Part model, mm, in its own coordinate system. A direction names the side the tool comes from. Give positions to 0.01 mm unless a question says otherwise; leave off trailing zeros. Write each loop counter-clockwise with the first axis right and the second up, starting at its lowest first coordinate (ties: lowest second). Pieces come first, ordered by that corner, then holes. Notation, with made-up numbers: M 69,15 L 81,15 A29 cw 81,48 Z; hole C -40,23 d11. An arc over 180 degrees is marked long. Use CSV: the item, a comma, the result in double quotes. Start each with the question number.
Item 1: Cut at A-A (z = 5). List the corners of the cut face in (x, y), then the cut area to 3 significant figures.
Item 2: Which spindle directions (+Z, -Z, +X, -X, +Y, -Y) get a long thin tool onto all of the face, cutting with end or side? Do faces 1 (the cylindrical face through (-69.244, -24.742, 7.365)), 2 (the flat face through (67, 46, 65.404)), 3 (the cylindrical face through (26.19, 75.94, 61.1)). Say none if no direction does.
Item 3: Drill centre lines: line 1 (X direction, y = 0, z = 48); line 2 (X direction, y = 0, z = -5); line 3 (Z direction, x = 64, y = 49). Where is each one in solid material? Low to high. Write a range as [from, to].
Item 4: Mould opens along Y. For faces 4 (the conical face through (-66.956, 31.627, -42.848)), 5 (the cylindrical face through (-60.5, -22, 61.2)), 6 (the flat face through (9, -77, -45.591)) say: released by +Y, released by -Y, zero draft, split by the parting line, or undercut.
Item 5: Pin check, flat tips, straight feed: pin 1 (2 mm diameter, centred on y = 47, z = 33, fed in from -X); pin 2 (1.5 mm diameter, centred on x = 30.5, y = -52, fed in from -Z); pin 3 (1.5 mm diameter, centred on y = -53, z = 11.5, fed in from +X). Stop position of each tip, or through.
from build123d import *

# Parameters (mm, degrees)
F2_T            = 4.5
F4_DEPTH        = 2.5
F4_COPIES_COUNT = 4
F5_S5_R         = 5
F5_T6_DEPTH     = 125
F5_S7_R         = 5
F5_T8_DEPTH     = 125
F5_S9_R         = 5
F5_T10_DEPTH    = 125
F5_S11_R        = 5
F5_T12_DEPTH    = 125


# Not quite as in the source:
# - a fillet or chamfer that OpenCascade refuses, or shapes differently, is made with other operations: its cross-section is extruded or revolved along the edge and cut away or added
# - a pattern or mirror of a feature is missing from the dataset's text; its kind, count and spacing are read off the source's solid
# - a shell that OpenCascade refuses in one call is made with other operations: the cavity is built on its own and cut out


with BuildPart() as f1:
    # F0 (on Front) → F1 (revolve)
    with BuildSketch(Plane.XZ):
        Polygon((9.3241020494, -43.0905388618), (9.3241020494, 56.9094611382), (-63.8827484445, 56.9094611382), (-63.8827484445, 65.4041709328), (-68.4650088725, 65.4041709328), (-68.4650088725, 56.9094611382), (-73.0472693004, 56.9094611382), (-73.0472693004, 61.1568160355), (-75.6501782344, 61.1568160355), (-78.0099242383, 55.0157746972), (-78.0099242383, 40.8573164567), (-73.0472693004, 36.7660618934), (-73.0472693004, -21.2237248131), (-78.0099242383, -30.2868788943), (-78.0099242383, -43.0905388618), align=None)
    revolve(axis=Axis((9.3241020494, 0, 6.9094611382), (0, 0, 1)))

    # F2: shell of thickness 4.5, made by hand


with BuildPart() as f2_core1:
    # F2_t2: copy of F1
    add(f1.part)

    # the walls: a layer under each face that stays
    f2_faces = [f2_core1.faces().sort_by_distance(p)[0] for p in [
        (82.5309525433, 0, 61.1568160355),
        (-42.5353052318, 51.8594072813, 65.4041709328),
        (87.1132129713, 0, 61.1568160355),
        (-67.5558445438, 21.9656990266, 56.9094611382),
        (91.6954733993, 0, 59.0331385869),
        (-69.9852262155, 22.6598080757, 61.1568160355),
        (95.4782553352, 0, 58.0862953663),
        (96.6581283371, 0, 47.936545577),
        (94.1768008682, 0, 38.8116891751),
        (91.6954733993, 0, 7.7711685402),
        (94.1768008682, 0, -25.7553018537),
        (96.6581283371, 0, -36.688708878),
        (9.3241020494, 0, -43.0905388618),
    ]]
    thicken(f2_faces, amount=-F2_T, mode=Mode.SUBTRACT)

    # F2_s3 → F2_t4 (revolve, cut)
    with BuildSketch(Plane.XZ):
        Polygon((-68.5100088725, 56.9544611382), (-63.9650088725, 56.9094611382), (-63.9650088725, 52.4094611382), (-68.4650088725, 52.4094611382), align=None)
    revolve(axis=Axis((9.3241020494, 0, 56.9094611382), (0, 0, 1)), mode=Mode.SUBTRACT)

    # F2_s5 → F2_t6 (revolve, cut)
    with BuildSketch(Plane.XZ):
        Polygon((-73.0022693004, 56.9544611382), (-73.0472693004, 52.4094611382), (-77.5472693004, 52.4094611382), (-77.5472693004, 56.9094611382), align=None)
    revolve(axis=Axis((9.3241020494, 0, 56.9094611382), (0, 0, 1)), mode=Mode.SUBTRACT)

    # F2_s7 → F2_t8 (revolve, cut)
    with BuildSketch(Plane.XZ):
        Polygon((-73.1208943097, 36.731340015), (-70.1847683719, 40.2382497389), (-68.5472693004, 38.8882817011), (-68.5472693004, 36.7660618934), align=None)
    revolve(axis=Axis((9.3241020494, 0, 36.7660618934), (0, 0, 1)), mode=Mode.SUBTRACT)

    # F2_s9 → F2_t10 (revolve, cut)
    with BuildSketch(Plane.XZ):
        Polygon((-73.1317395514, -21.2021123331), (-68.5472693004, -21.2237248131), (-68.5472693004, -22.375090633), (-69.1002442047, -23.3849728075), align=None)
    revolve(axis=Axis((9.3241020494, 0, -21.2237248131), (0, 0, 1)), mode=Mode.SUBTRACT)


with BuildPart() as f1_1:
    add(f1.part)

    # what is left inside the walls is the cavity
    f2_cavity = [f2_core1.part.solids().sort_by_distance(p)[0] for p in [
        (87.150473, 0, 18.467158),
    ]]
    add(f2_cavity, mode=Mode.SUBTRACT)

    # F3 (on face) → F4 (join)
    with BuildSketch(Plane(origin=(0, 0, -43.0905388618), x_dir=(1, 0, 0), z_dir=(0, 0, -1))):
        with BuildLine():
            ThreePointArc((9.3241020494, 77.3856560126), (11.8241020494, 77.3452633101), (14.3214922181, 77.2241273697))
            ThreePointArc((14.3214922181, 77.2241273697), (14.323449549, 77.30488115), (14.3241020494, 77.3856560126))
            ThreePointArc((14.3241020494, 77.3856560126), (12.8596359554, 80.9211899185), (9.3241020494, 82.3856560126))
            Line((9.3241020494, 82.3856560126), (9.3241020494, 77.3856560126))
        make_face()
        with BuildLine():
            Line((9.3241020494, 77.3856560126), (9.3241020494, 72.3856560126))
            ThreePointArc((9.3241020494, 72.3856560126), (12.8020581148, 73.7934670411), (14.3214922181, 77.2241273697))
            ThreePointArc((14.3214922181, 77.2241273697), (11.8241020494, 77.3452633101), (9.3241020494, 77.3856560126))
        make_face()
        with BuildLine():
            ThreePointArc((4.3267118808, 77.2241273697), (5.8461459841, 73.7934670411), (9.3241020494, 72.3856560126))
            Line((9.3241020494, 72.3856560126), (9.3241020494, 77.3856560126))
            ThreePointArc((9.3241020494, 77.3856560126), (6.8241020494, 77.3452633101), (4.3267118808, 77.2241273697))
        make_face()
        with BuildLine():
            ThreePointArc((9.3241020494, 82.3856560126), (5.7319130779, 80.863612078), (4.3267118808, 77.2241273697))
            ThreePointArc((4.3267118808, 77.2241273697), (6.8241020494, 77.3452633101), (9.3241020494, 77.3856560126))
            Line((9.3241020494, 77.3856560126), (9.3241020494, 82.3856560126))
        make_face()
    f4 = extrude(amount=F4_DEPTH)

    # F4_copies: F4 ×4 about axis
    f4_copies_axis = Axis((9.324102, 0, 0), (0, 0, 1))
    for i in range(1, F4_COPIES_COUNT):
        add(f4.rotate(f4_copies_axis, i * 360 / F4_COPIES_COUNT))

    # F5: chamfer of 5 on 1 edges, made by hand


with BuildPart() as f5_tool2:
    # F5_s3 → F5_t4 (revolve)
    with BuildSketch(Plane.XZ):
        Polygon((-78.0099242383, -38.0905388618), (-73.0099242383, -43.0905388618), (-78.0099242383, -43.0905388618), align=None)
    revolve(axis=Axis((9.3241020494, 0, -43.0905388618), (0, 0, 1)))

    # F5_s5 → F5_t6 (cut, symmetric)
    with BuildSketch(Plane.XY.offset(-40.6)):
        with Locations((86.7097580126, 4.94e-08)):
            Circle(F5_S5_R)
    extrude(amount=F5_T6_DEPTH, both=True, mode=Mode.SUBTRACT)

    # F5_s7 → F5_t8 (cut, symmetric)
    with BuildSketch(Plane.XY.offset(-40.6)):
        with Locations((9.3241019506, 77.3856560126)):
            Circle(F5_S7_R)
    extrude(amount=F5_T8_DEPTH, both=True, mode=Mode.SUBTRACT)

    # F5_s9 → F5_t10 (cut, symmetric)
    with BuildSketch(Plane.XY.offset(-40.6)):
        with Locations((9.3241020494, -77.3856560126)):
            Circle(F5_S9_R)
    extrude(amount=F5_T10_DEPTH, both=True, mode=Mode.SUBTRACT)

    # F5_s11 → F5_t12 (cut, symmetric)
    with BuildSketch(Plane.XY.offset(-40.6)):
        with Locations((-68.0615540126, -4.94e-08)):
            Circle(F5_S11_R)
    extrude(amount=F5_T12_DEPTH, both=True, mode=Mode.SUBTRACT)


with BuildPart() as f1_2:
    add(f1_1.part)

    # F5_t1: cut F5_tool2
    add(f5_tool2.part, mode=Mode.SUBTRACT)


solid = f1_2.part
Worked answers:
1,outline,"C 9.32,0 d164.74; hole C 9.32,0 d155.74"
1,area,"2,270 mm^2"
2,face 1,"none"
2,face 2,"+Z, +X, -X, +Y, -Y"
2,face 3,"+Z"
3,line 1,"x = [-78.01, -73.51], [92.16, 96.66]"
3,line 2,"x = [-73.05, -68.55], [87.2, 91.7]"
3,line 3,"z = [-43.09, -38.59], [52.41, 65.4]"
4,face 4,"split by the parting line"
4,face 5,"undercut"
4,face 6,"zero draft"
5,pin 1,"stops at x = -59.01"
5,pin 2,"stops at z = -43.09"
5,pin 3,"stops at x = 73"
